Design review of the part built by this model. Coordinates are the model's own, in mm. Face numbers are marked on the shaded views. A direction names the side the tool comes from. Coordinates: 2 decimals unless noted, no trailing zeros. Write each loop counter-clockwise with the first axis right and the second up, starting at its lowest first coordinate (ties: lowest second). Pieces come first, ordered by that corner, then holes. Notation, with made-up numbers: (63, -25) - (76, -25) arc R22 ccw to (76, -13) - close; hole circle Ø7 at (46.5, 69). An arc over 180 degrees is marked (long way). Answer as a JSON object with one key per item and string values.
```python
from build123d import *

# Parameters (mm, degrees)
SKETCH1_R           = 1.6
BOSS_EXTRUDE1_DEPTH = 3.2
SKETCH2_W           = 30
SKETCH2_H           = 3
BOSS_EXTRUDE2_DEPTH = 8
SKETCH3_R           = 1.6
CUT_EXTRUDE1_DEPTH  = 25.960610678
FILLET1_R           = 0.5
CHAMFER1_SIZE       = 1


with BuildPart() as part:
    # Sketch1 → Boss-Extrude1 (new body)
    with BuildSketch(Plane.XY):
        with BuildLine():
            Line((-15, -3), (15, -3))
            Line((15, -3), (15, 12))
            ThreePointArc((15, 12), (10.489637029, 16.510362971), (5.979274058, 12))
            Line((5.979274058, 12), (8, 8.5))
            Line((8, 8.5), (8, 0))
            Line((8, 0), (-8, 0))
            Line((-8, 0), (-8, 8.5))
            Line((-8, 8.5), (-5.979274058, 12))
            ThreePointArc((-5.979274058, 12), (-10.489637029, 16.510362971), (-15, 12))
            Line((-15, 12), (-15, -3))
        make_face()
        with Locations((-10, 12)):
            Circle(SKETCH1_R, mode=Mode.SUBTRACT)
        with Locations((10, 12)):
            Circle(SKETCH1_R, mode=Mode.SUBTRACT)
    extrude(amount=BOSS_EXTRUDE1_DEPTH)

    # Sketch2 → Boss-Extrude2 (add)
    with BuildSketch(Plane.XY.offset(3.2)):
        with Locations((0, -1.5)):
            Rectangle(SKETCH2_W, SKETCH2_H)
    extrude(amount=BOSS_EXTRUDE2_DEPTH)

    # Sketch3 → Cut-Extrude1 (cut, through all)
    with BuildSketch(Plane(origin=(0, 0, 0), x_dir=(1, 0, 0), z_dir=(0, 1, 0))):
        with Locations(Location((-10, -7.2, 0), (0, 0, 270))):
            Circle(SKETCH3_R)
        with Locations(Location((10, -7.2, 0), (0, 0, 270))):
            Circle(SKETCH3_R)
    extrude(amount=-CUT_EXTRUDE1_DEPTH, mode=Mode.SUBTRACT)

    # Fillet1
    fillet1_edges = [part.edges().sort_by_distance(p)[0] for p in [
        (8, 4.25, 0),
        (6.989637029, 10.25, 0),
        (10.489637029, 16.510362971, 0),
        (15, 4.5, 0),
        (-15, 4.5, 0),
        (-10.489637029, 16.510362971, 0),
        (10.489637029, 16.510362971, 3.2),
        (6.989637029, 10.25, 3.2),
        (8, 4.25, 3.2),
        (-8, 4.25, 3.2),
        (-6.989637029, 10.25, 3.2),
        (15, 6, 3.2),
        (-10.489637029, 16.510362971, 3.2),
        (-15, -1.5, 11.2),
        (15, -1.5, 11.2),
        (-15, 6, 3.2),
        (-6.989637029, 10.25, 0),
        (-8, 4.25, 0),
    ]]
    fillet(fillet1_edges, radius=FILLET1_R)

    # Chamfer1
    # the kernel refuses this chamfer: 1 mm, written as the material it adds along each edge
    with BuildSketch(Plane(origin=(-8.5, 0, 3.2), x_dir=(0, 0.9996219169112968, -0.027495876610586494), z_dir=(-1, 0, 0)), Plane(origin=(14.5, 0, 3.2), x_dir=(0, 0.9996219169112968, -0.027495876610586494), z_dir=(-1, 0, 0))) as chamfer1_piece_1:
        Polygon((CHAMFER1_SIZE * 0.999621916911, -CHAMFER1_SIZE * 0.0274958766106), (-CHAMFER1_SIZE * 0.0274958766106, -CHAMFER1_SIZE * 0.999621916911), (0, 0), align=None)
    extrude(amount=6)
    with BuildSketch(Plane(origin=(-8, 0, 0.5), x_dir=(-0.02749587661058563, 0.9996219169112968, 0), z_dir=(0, 0, 1))) as chamfer1_piece_2:
        Polygon((CHAMFER1_SIZE * 0.999621916911, -CHAMFER1_SIZE * 0.0274958766106), (-CHAMFER1_SIZE * 0.0274958766106, -CHAMFER1_SIZE * 0.999621916911), (0, 0), align=None)
    extrude(amount=2.2)
    with BuildSketch(Plane(origin=(8, 0, 0.5), x_dir=(0.027495876610585633, 0.9996219169112968, 0), z_dir=(0, 0, 1))) as chamfer1_piece_3:
        Polygon((CHAMFER1_SIZE * 0.999621916911, CHAMFER1_SIZE * 0.0274958766106), (-CHAMFER1_SIZE * 0.0274958766106, CHAMFER1_SIZE * 0.999621916911), (0, 0), align=None)
    extrude(amount=2.2)
    with BuildSketch(Plane(origin=(-14.5, 0, 2.7), x_dir=(0.006283143965557512, 0, 0.9999802608561372), z_dir=(-0.9999802608561372, 0, 0.006283143965557512))) as chamfer1_piece_4_section:
        Polygon((-0.5 - CHAMFER1_SIZE, 0), (-0.5, CHAMFER1_SIZE), (-0.5, 0), align=None)
    chamfer1_piece_4 = revolve(axis=Axis((-14.5, 0, 2.7), (0, 1, 0)), revolution_arc=359.64, mode=Mode.PRIVATE)
    chamfer1_piece_4 = split(chamfer1_piece_4, bisect_by=Plane(origin=(-15, 0.469782675, 3.086220861), z_dir=(1, 0, 0)), keep=Keep.TOP, mode=Mode.PRIVATE)
    add(chamfer1_piece_4)
    with BuildSketch(Plane(origin=(-8.5, 0, 0.5), x_dir=(0.9999802608561372, 0, 0.006283143965558622), z_dir=(0.006283143965558622, 0, -0.9999802608561372))) as chamfer1_piece_5_section:
        Polygon((-0.5, -CHAMFER1_SIZE), (-0.5 - CHAMFER1_SIZE, 0), (-0.5, 0), align=None)
    chamfer1_piece_5 = revolve(axis=Axis((-8.5, 0, 0.5), (0, -1, 0)), revolution_arc=359.64, mode=Mode.PRIVATE)
    chamfer1_piece_5 = split(chamfer1_piece_5, bisect_by=Plane(origin=(-8.113779143, 0.469782674, 0), z_dir=(0, 0, 1)), keep=Keep.TOP, mode=Mode.PRIVATE)
    add(chamfer1_piece_5)
    with BuildSketch(Plane(origin=(8.5, 0, 2.7), x_dir=(-1, 0, 0), z_dir=(0, 0, -1))) as chamfer1_piece_6:
        Polygon((0.5, CHAMFER1_SIZE), (0.5 + CHAMFER1_SIZE, 0), (0.5, 0), align=None)
    revolve(axis=Axis((8.5, 0, 2.7), (0, 1, 0)), revolution_arc=90)
    with BuildSketch(Plane(origin=(8.5, 0, 0.5), x_dir=(-0.9999802608561372, 0, 0.006283143965558622), z_dir=(-0.006283143965558622, 0, -0.9999802608561372))) as chamfer1_piece_7_section:
        Polygon((-0.5, CHAMFER1_SIZE), (-0.5 - CHAMFER1_SIZE, 0), (-0.5, 0), align=None)
    chamfer1_piece_7 = revolve(axis=Axis((8.5, 0, 0.5), (0, 1, 0)), revolution_arc=359.64, mode=Mode.PRIVATE)
    chamfer1_piece_7 = split(chamfer1_piece_7, bisect_by=Plane(origin=(8.113779139, 0.469782675, 0), z_dir=(0, 0, 1)), keep=Keep.TOP, mode=Mode.PRIVATE)
    add(chamfer1_piece_7)
    with BuildSketch(Plane(origin=(14.5, 0, 2.7), x_dir=(0, 0, 1), z_dir=(-1, 0, 0))) as chamfer1_piece_8_section:
        Polygon((0.5, CHAMFER1_SIZE), (0.5 + CHAMFER1_SIZE, 0), (0.5, 0), align=None)
    chamfer1_piece_8 = revolve(axis=Axis((14.5, 0, 2.7), (0, 1, 0)), revolution_arc=359.64, mode=Mode.PRIVATE)
    chamfer1_piece_8 = split(chamfer1_piece_8, bisect_by=Plane(origin=(15, 0.469782675, 3.086220861), z_dir=(-1, 0, 0)), keep=Keep.TOP, mode=Mode.PRIVATE)
    add(chamfer1_piece_8)
    with BuildSketch(Plane(origin=(-8.5, 0, 2.7), x_dir=(0, 0, 1), z_dir=(-1, 0, 0))) as chamfer1_piece_9:
        Polygon((0.5, CHAMFER1_SIZE), (0.5 + CHAMFER1_SIZE, 0), (0.5, 0), align=None)
    revolve(axis=Axis((-8.5, 0, 2.7), (0, 1, 0)), revolution_arc=90)


solid = part.part
```
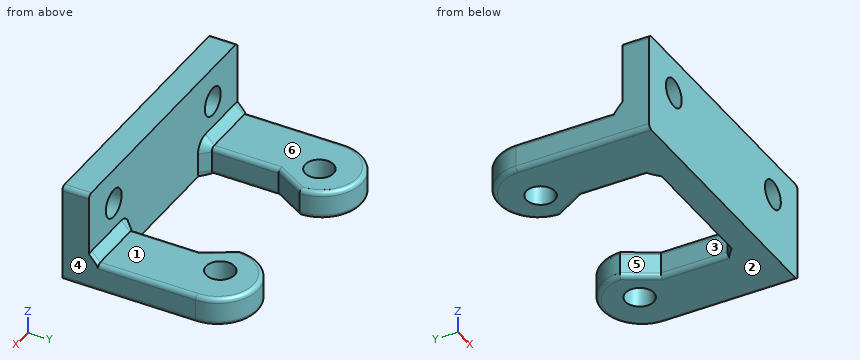
(1) The part is to be moulded in two halves that separate along X. For the marked faces 4, 5 and 6, say which applies: pulls with the +X half, pulls with the -X half, needs draft (parallel to the pull), parting line crosses it, or undercut.
Solved:
{"face 4": "pulls with the +X half", "face 5": "undercut", "face 6": "needs draft"}
(2) Take a section at A-A, the plane z = 7.2. Write out the cut boundary in (x, y), and give its area (3 significant figures).
Solved:
{"outline": "(-15, -3) - (-11.6, -3) - (-11.6, 0) - (-15, 0) - close; (-8.4, -3) - (8.4, -3) - (8.4, 0) - (-8.4, 0) - close; (11.6, -3) - (15, -3) - (15, 0) - (11.6, 0) - close", "area": "70.8 mm^2"}
(3) To check wall thickness, follow line 1 (X direction, y = -1.4, z = 7.2); line 2 (Y direction, x = -11.5, z = 6.5); line 3 (X direction, y = 11.75, z = 0.5). State the ranges of each line that lie inside material, in increasing order. Write a range as from..to.
Solved:
{"line 1": "x = -15..-11.6, -8.4..8.4, 11.6..15", "line 2": "y = -3..0", "line 3": "x = -15..-11.58, -8.42..-6.12, 6.12..8.42, 11.58..15"}
(4) For pin 1 (2.5 mm diameter, centred on x = 10, y = 12, fed in from -Z); pin 2 (9 mm diameter, centred on x = -9.5, y = 10.5, fed in from +Z); pin 3 (5.5 mm diameter, centred on x = 0.5, z = 4, fed in from +Y), all flat-tipped, find the tip position at first contact; note any pin that passes through.
Solved:
{"pin 1": "passes through", "pin 2": "stops at z = 3.2", "pin 3": "stops at y = 0"}
(5) Take a section at D-D, the plane z = 5. Write out the cut boundary in (x, y).
Solved:
{"outline": "(-15, -3) - (15, -3) - (15, 0) - (-15, 0) - close"}
(6) Tool access review of the marked faces 1, 2 and 3: name each direction out of +Z, -Z, +X, -X, +Y, -Y from which nothing blocks a thin tool from reaching the whole face with its end or side.
Solved:
{"face 1": "+Z, +X, -X, +Y", "face 2": "-Z, +X, -X, +Y, -Y", "face 3": "+Z, -Z"}
(7) Take a section at C-C, the plane x = 0.5. Write out the cut boundary in (y, z).
Solved:
{"outline": "(-3, 0) - (0, 0) - (0, 11.2) - (-3, 11.2) - close"}
(8) Take a section at B-B, the plane y = 2.75. Write out the cut boundary in (x, z).
Solved:
{"outline": "(-15, 0.5) arc R0.5 ccw to (-14.5, 0) - (-8.5, 0) arc R0.5 ccw to (-8, 0.5) - (-8, 2.7) arc R0.5 ccw to (-8.5, 3.2) - (-14.5, 3.2) arc R0.5 ccw to (-15, 2.7) - close; (8, 0.5) arc R0.5 ccw to (8.5, 0) - (14.5, 0) arc R0.5 ccw to (15, 0.5) - (15, 2.7) arc R0.5 ccw to (14.5, 3.2) - (8.5, 3.2) arc R0.5 ccw to (8, 2.7) - close"}
